```python
from build123d import *

# Parameters (mm, degrees)
F0_W     = 20
F0_H     = 32
F0_R     = 3.75
F1_DEPTH = 2
F2_DEPTH = 10
F4_DEPTH = 4


with BuildPart() as f1:
    # F0 (on Top) → F1 (new body)
    with BuildSketch(Plane.XY):
        Polygon((12, 18), (4, 18), (-4, 18), (-12, 18), (-12, 2), (-12, -2), (-12, -18), (-4, -18), (4, -18), (12, -18), (12, -2), (12, 2), align=None)
        Rectangle(F0_W, F0_H, mode=Mode.SUBTRACT)
        Rectangle(F0_W, F0_H)
        with BuildLine():
            Line((-12, 18), (-4, 18))
            Line((-4, 18), (-25, 32.8394541729))
            ThreePointArc((-25, 32.8394541729), (-24.4406610105, 31.4684175156), (-24.25, 30))
            ThreePointArc((-24.25, 30), (-27.9074485781, 24.6442807629), (-34.2269490597, 26.1018720331))
            Line((-34.2269490597, 26.1018720331), (-12, 2))
            Line((-12, 2), (-12, 18))
        make_face()
        with BuildLine():
            ThreePointArc((34.2269490597, 26.1018720331), (26.6091070185, 25.3562574589), (25, 32.8394541729))
            Line((25, 32.8394541729), (4, 18))
            Line((4, 18), (12, 18))
            Line((12, 18), (12, 2))
            Line((12, 2), (34.2269490597, 26.1018720331))
        make_face()
        with BuildLine():
            Line((-12, -18), (-12, -2))
            Line((-12, -2), (-34.2269490597, -26.1018720331))
            ThreePointArc((-34.2269490597, -26.1018720331), (-27.9074485781, -24.6442807629), (-24.25, -30))
            ThreePointArc((-24.25, -30), (-24.4406610105, -31.4684175156), (-25, -32.8394541729))
            Line((-25, -32.8394541729), (-4, -18))
            Line((-4, -18), (-12, -18))
        make_face()
        with BuildLine():
            Line((34.2269490597, -26.1018720331), (12, -2))
            Line((12, -2), (12, -18))
            Line((12, -18), (4, -18))
            Line((4, -18), (25, -32.8394541729))
            ThreePointArc((25, -32.8394541729), (26.6091070185, -25.3562574589), (34.2269490597, -26.1018720331))
        make_face()
        with BuildLine():
            ThreePointArc((-24.25, 30), (-24.4406610105, 31.4684175156), (-25, 32.8394541729))
            ThreePointArc((-25, 32.8394541729), (-33.3908929815, 34.6437425411), (-34.2269490597, 26.1018720331))
            ThreePointArc((-34.2269490597, 26.1018720331), (-27.9074485781, 24.6442807629), (-24.25, 30))
        make_face()
        with Locations((-30, 30)):
            Circle(F0_R, mode=Mode.SUBTRACT)
        with BuildLine():
            ThreePointArc((35.75, -30), (35.3557192371, -27.9074485781), (34.2269490597, -26.1018720331))
            ThreePointArc((34.2269490597, -26.1018720331), (26.6091070185, -25.3562574589), (25, -32.8394541729))
            ThreePointArc((25, -32.8394541729), (31.4684175156, -35.5593389895), (35.75, -30))
        make_face()
        with Locations((30, -30)):
            Circle(F0_R, mode=Mode.SUBTRACT)
        with BuildLine():
            ThreePointArc((34.2269490597, 26.1018720331), (35.3557192371, 27.9074485781), (35.75, 30))
            ThreePointArc((35.75, 30), (31.4684175156, 35.5593389895), (25, 32.8394541729))
            ThreePointArc((25, 32.8394541729), (26.6091070185, 25.3562574589), (34.2269490597, 26.1018720331))
        make_face()
        with Locations((30, 30)):
            Circle(F0_R, mode=Mode.SUBTRACT)
        with BuildLine():
            ThreePointArc((-24.25, -30), (-27.9074485781, -24.6442807629), (-34.2269490597, -26.1018720331))
            ThreePointArc((-34.2269490597, -26.1018720331), (-33.3908929815, -34.6437425411), (-25, -32.8394541729))
            ThreePointArc((-25, -32.8394541729), (-24.4406610105, -31.4684175156), (-24.25, -30))
        make_face()
        with Locations((-30, -30)):
            Circle(F0_R, mode=Mode.SUBTRACT)
    extrude(amount=F1_DEPTH)

    # F0 (on Top) → F2 (join)
    with BuildSketch(Plane.XY):
        with BuildLine():
            ThreePointArc((-24.25, -30), (-27.9074485781, -24.6442807629), (-34.2269490597, -26.1018720331))
            ThreePointArc((-34.2269490597, -26.1018720331), (-33.3908929815, -34.6437425411), (-25, -32.8394541729))
            ThreePointArc((-25, -32.8394541729), (-24.4406610105, -31.4684175156), (-24.25, -30))
        make_face()
        with Locations((-30, -30)):
            Circle(F0_R, mode=Mode.SUBTRACT)
        with BuildLine():
            ThreePointArc((35.75, -30), (35.3557192371, -27.9074485781), (34.2269490597, -26.1018720331))
            ThreePointArc((34.2269490597, -26.1018720331), (26.6091070185, -25.3562574589), (25, -32.8394541729))
            ThreePointArc((25, -32.8394541729), (31.4684175156, -35.5593389895), (35.75, -30))
        make_face()
        with Locations((30, -30)):
            Circle(F0_R, mode=Mode.SUBTRACT)
        with BuildLine():
            ThreePointArc((34.2269490597, 26.1018720331), (35.3557192371, 27.9074485781), (35.75, 30))
            ThreePointArc((35.75, 30), (31.4684175156, 35.5593389895), (25, 32.8394541729))
            ThreePointArc((25, 32.8394541729), (26.6091070185, 25.3562574589), (34.2269490597, 26.1018720331))
        make_face()
        with Locations((30, 30)):
            Circle(F0_R, mode=Mode.SUBTRACT)
        with BuildLine():
            ThreePointArc((-24.25, 30), (-24.4406610105, 31.4684175156), (-25, 32.8394541729))
            ThreePointArc((-25, 32.8394541729), (-33.3908929815, 34.6437425411), (-34.2269490597, 26.1018720331))
            ThreePointArc((-34.2269490597, 26.1018720331), (-27.9074485781, 24.6442807629), (-24.25, 30))
        make_face()
        with Locations((-30, 30)):
            Circle(F0_R, mode=Mode.SUBTRACT)
    extrude(amount=F2_DEPTH)

    # F0 (on Top) → F4 (join)
    with BuildSketch(Plane.XY):
        Polygon((12, 18), (4, 18), (-4, 18), (-12, 18), (-12, 2), (-12, -2), (-12, -18), (-4, -18), (4, -18), (12, -18), (12, -2), (12, 2), align=None)
        Rectangle(F0_W, F0_H, mode=Mode.SUBTRACT)
    extrude(amount=F4_DEPTH)


solid = f1.part
```
Source: CAD feature listing. Evaluate the final solid. Frame: model axes, mm. A direction names the side the tool comes from. Round coordinates to 2 decimals unless told otherwise and drop trailing zeros. Order: outer loops, then holes, each group sorted by start corner. A loop starts at its lowest first (then second) coordinate and runs counter-clockwise, first axis right, second up. Notation, with made-up numbers: (78.25, -28) -> (109.25, -28) arc R19 ccw to (109.25, 1) -> close; hole circle Ø4 at (80, -39). An arc over 180 degrees is marked (long way). One line per item, written item: value. Start each with the question number.
Q1. Access query for faces 4 (the flat face through (23.27, -14.22, 0.99)), 5 (the flat face through (0, -18, 2)), 6 (the flat face through (-10, 0, 3)), 7 (the flat face through (-12, 0, 3)). Directions: +Z, -Z, +X, -X, +Y, -Y. A direction counts if a zero-diameter tool reaches every point of the face in a straight line with its end or side. Return the directions, or none.
Q2. Section query C-C (x = -19.5). Return the cut outline in (y, z).
Q3. Draft query along X for faces 1 (the flat face through (-11, 1, 4)), 2 (the flat face through (22.958, 13.882, 0.986)), 3 (the flat face through (18, 19, 2)). Return one class per face: pulls with the +X half, pulls with the -X half, needs draft (parallel to the pull), parting line crosses it, or undercut.
Q4. Section query A-A (z = 5.5). Return the cut outline in (x, y), plus the area to 3 significant figures.
Q5. Section query D-D (y = 19.5). Return the cut outline in (x, z).
Q6. Section query B-B (y = 30). Return the cut outline in (x, z).
Q7. Pin query (flat end, axial travel): pin 1 (9 mm diameter, centred on x = -23.5, y = 18.5, fed in from +Z); pin 2 (1 mm diameter, centred on y = -7, z = 5, fed in from -X); pin 3 (4.5 mm diameter, centred on y = 1.5, z = 2.5, fed in from +X); pin 4 (2 mm diameter, centred on x = -4, z = 2.5, fed in from +Y). Return the tip coordinate at first contact, or that it passes through.
Q8. Material intervals for probe 1 along Y at (x, z) = (-30, 2.75); probe 2 along X at (y, z) = (-14, 2.75); probe 3 along Z at (x, y) = (20, 27.5), sorted ascending.
Findings below:
1. face 4: +Z, -Z, +X
1. face 5: +Z, -Y
1. face 6: +Z
1. face 7: +Z, -X
2. outline: (-28.95, 0) -> (-10.13, 0) -> (-10.13, 2) -> (-28.95, 2) -> close; (10.13, 0) -> (28.95, 0) -> (28.95, 2) -> (10.13, 2) -> close
3. face 1: needs draft
3. face 2: pulls with the +X half
3. face 3: undercut
4. outline: circle Ø11.5 at (-30, -30); circle Ø11.5 at (-30, 30); circle Ø11.5 at (30, -30); circle Ø11.5 at (30, 30); hole circle Ø7.5 at (-30, -30); hole circle Ø7.5 at (-30, 30); hole circle Ø7.5 at (30, -30); hole circle Ø7.5 at (30, 30)
4. area: 239 mm²
5. outline: (-28.14, 0) -> (-6.12, 0) -> (-6.12, 2) -> (-28.14, 2) -> close; (6.12, 0) -> (28.14, 0) -> (28.14, 2) -> (6.12, 2) -> close
6. outline: (-35.75, 0) -> (-33.75, 0) -> (-33.75, 10) -> (-35.75, 10) -> close; (-26.25, 0) -> (-20.98, 0) -> (-20.98, 2) -> (-24.25, 2) -> (-24.25, 10) -> (-26.25, 10) -> close; (20.98, 0) -> (26.25, 0) -> (26.25, 10) -> (24.25, 10) -> (24.25, 2) -> (20.98, 2) -> close; (33.75, 0) -> (35.75, 0) -> (35.75, 10) -> (33.75, 10) -> close
7. pin 1: z = 2
7. pin 2: through
7. pin 3: x = 13.56
7. pin 4: y = 18.61
8. probe 1: -35.75 to -33.75, -26.25 to -24.25, 24.25 to 26.25, 33.75 to 35.75
8. probe 2: -12 to -10, 10 to 12
8. probe 3: 0 to 2
